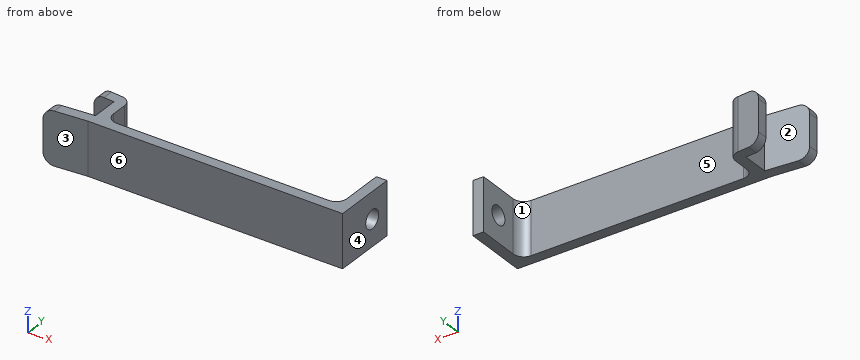
from build123d import *

# Parameters (mm, degrees)
F1_DEPTH = 10
F2_R     = 2
F4_D     = 3.5
F4_DEPTH = 2.001


with BuildPart() as f1:
    # F0 (on Top) → F1 (new body)
    with BuildSketch(Plane.XY):
        Polygon((0, 0), (48, 0), (48, 12), (46, 12), (46, 2), (2, 2), (2, 8.8250226729), (-4, 9.3499546541), (-4, 7.3499546541), (0, 7), (0, 2), (-8, 1.3000906918), (-8, -0.6999093082), align=None)
    extrude(amount=F1_DEPTH)

    # F2
    f2_edges = [f1.edges().sort_by_distance(p)[0] for p in [
        (-8, 0.300091, 10),
        (-8, 0.300091, 0),
        (-4, 8.349955, 0),
        (-4, 8.349955, 10),
        (2, 2, 5),
        (2, 8.825023, 5),
        (46, 2, 5),
    ]]
    fillet(f2_edges, radius=F2_R)

    # F4 (through all, one way)
    with BuildSketch(Plane(origin=(46, 0, 0), x_dir=(0, -1, 0), z_dir=(-1, 0, 0))):
        with Locations((-8, 5)):
            Circle(F4_D / 2)
    extrude(amount=-F4_DEPTH, mode=Mode.SUBTRACT)


solid = f1.part
Source: CAD feature listing. Evaluate the final solid. Frame: model axes, mm. Face numbers are marked on the shaded views. A direction names the side the tool comes from. Round coordinates to 2 decimals unless told otherwise and drop trailing zeros. Loops run counter-clockwise (first coordinate to the right, second up) from the corner with the lowest first, then second, coordinate; pieces in that order, holes last. Notation, with made-up numbers: (80, 62.5) -> (131, 62.5) arc R13 cw to (131, 71.5) -> close; hole circle Ø11 at (71.5, 56.25). An arc over 180 degrees is marked (long way). Answer as a JSON object with one key per item and string values. Group by question number.
Q1. Mould query, pull axis X, two halves, no side actions, for the marked faces 4, 5 and 6. Classes: pulls with the +X half, pulls with the -X half, needs draft (parallel to the pull), parting line crosses it, or undercut.
Q2. Access query for the marked faces 1, 2 and 3. Directions: +Z, -Z, +X, -X, +Y, -Y. A direction counts if a zero-diameter tool reaches every point of the face in a straight line with its end or side. Return the directions, or none.
Q3. Section query B-B (x = -3.5). Output: boundary loops of the cut face in (y, z), plus the area to 3 significant figures.
Q4. Section query A-A (z = 5). Output: boundary loops of the cut face in (x, y), plus the area to 3 significant figures.
Q5. Section query C-C (y = 3.5). Output: boundary loops of the cut face in (x, z), plus the area to 3 significant figures.
Q6. Contact query for flat-ended pins moving along their axis: P1, Ø2.5, axis at y = 5, z = 5, coming from the -X side; P2, Ø1.6, axis at y = 8.5, z = 6.5, coming from the -X side; P3, Ø3, axis at x = 36, z = 2.5, coming from the +Y side. Output: stop coordinate, or through.
Q7. Section query D-D (y = 8). Output: boundary loops of the cut face in (x, z).
Q8. Ray query, line 1 (Z direction, x = 47.25, y = 8); line 2 (X direction, y = 6, z = 0.75); line 3 (Y direction, x = -1, z = 1). Return the intervals inside material, ascending. Write a range as from..to.
Completed:
{
 "1": {"face 4": "pulls with the +X half", "face 5": "undercut", "face 6": "needs draft"},
 "2": {"face 1": "+Z, -Z, +Y", "face 2": "+Z, -Z, -X", "face 3": "+Z, -Z, +X, -Y"},
 "3": {"outline": "(-0.31, 0) -> (1.69, 0) -> (1.69, 10) -> (-0.31, 10) -> close; (7.31, 0.68) -> (9.31, 0.68) -> (9.31, 9.32) -> (7.31, 9.32) -> close", "area": "37.3 mm²"},
 "4": {"outline": "(-8, -0.7) -> (0, 0) -> (48, 0) -> (48, 6.25) -> (46, 6.25) -> (46, 4) arc R2 cw to (44, 2) -> (4, 2) arc R2 cw to (2, 4) -> (2, 6.99) arc R2 ccw to (0.17, 8.98) -> (-4, 9.35) -> (-4, 7.35) -> (0, 7) -> (0, 2) -> (-8, 1.3) -> close; (46, 9.75) -> (48, 9.75) -> (48, 12) -> (46, 12) -> close", "area": "148 mm²"},
 "5": {"outline": "(0, 0) -> (2.06, 0) -> (2.06, 10) -> (0, 10) -> close; (45.94, 0) -> (48, 0) -> (48, 10) -> (45.94, 10) -> close", "area": "41.3 mm²"},
 "6": {"P1": "x = 0", "P2": "x = -4", "P3": "y = 2"},
 "7": {"outline": "(-4, 2) arc R2 ccw to (-2, 0) -> (1.73, 0) -> (1.73, 10) -> (-2, 10) arc R2 ccw to (-4, 8) -> close; (46, 0) -> (48, 0) -> (48, 3.25) -> (46, 3.25) -> close; (46, 6.75) -> (48, 6.75) -> (48, 10) -> (46, 10) -> close"},
 "8": {"line 1": "0..3.25, 6.75..10", "line 2": "0..2, 46..48", "line 3": "-0.09..1.91, 7.09..9.09"}
}
